from build123d import *

# Parameters (mm, degrees)
SKETCH1_W           = 45
SKETCH1_H           = 24
BOSS_EXTRUDE1_DEPTH = 9.3
SKETCH2_R           = 1.25
BOSS_EXTRUDE2_DEPTH = 9.3
SKETCH3_W           = 15
SKETCH3_H           = 24
BOSS_EXTRUDE3_DEPTH = 4.8
SKETCH4_W           = 11.1
SKETCH4_H           = 20.8
SKETCH4_R           = 0.75
CUT_EXTRUDE1_DEPTH  = 7


with BuildPart() as part:
    # Sketch1 → Boss-Extrude1 (new body)
    with BuildSketch(Plane(origin=(0, 0, 0), x_dir=(1, 0, 0), z_dir=(0, 1, 0))):
        with Locations((22.5, 12)):
            Rectangle(SKETCH1_W, SKETCH1_H)
    extrude(amount=BOSS_EXTRUDE1_DEPTH)

    # Sketch2 → Boss-Extrude2 (add)
    with BuildSketch(Plane(origin=(45, 0, 0), x_dir=(0, 0, -1), z_dir=(1, 0, 0))):
        with Locations((12, 2.083449871)):
            Circle(SKETCH2_R)
    extrude(amount=BOSS_EXTRUDE2_DEPTH)

    # Sketch3 → Boss-Extrude3 (add)
    with BuildSketch(Plane(origin=(0, 9.3, 0), x_dir=(1, 0, 0), z_dir=(0, 1, 0))):
        with Locations((7.5, 12)):
            Rectangle(SKETCH3_W, SKETCH3_H)
    extrude(amount=BOSS_EXTRUDE3_DEPTH)

    # Sketch4 → Cut-Extrude1 (cut)
    with BuildSketch(Plane(origin=(0, 14.1, 0), x_dir=(1, 0, 0), z_dir=(0, 1, 0))):
        with Locations((7.85, 12)):
            Rectangle(SKETCH4_W, SKETCH4_H)
        with Locations((4.85, 19.9)):
            Circle(SKETCH4_R, mode=Mode.SUBTRACT)
        with Locations((7.85, 19.9)):
            Circle(SKETCH4_R, mode=Mode.SUBTRACT)
        with Locations((10.85, 19.9)):
            Circle(SKETCH4_R, mode=Mode.SUBTRACT)
        with Locations((4.85, 17.3)):
            Circle(SKETCH4_R, mode=Mode.SUBTRACT)
        with Locations((7.85, 17.3)):
            Circle(SKETCH4_R, mode=Mode.SUBTRACT)
        with Locations((10.85, 17.3)):
            Circle(SKETCH4_R, mode=Mode.SUBTRACT)
        with Locations((4.85, 14.7)):
            Circle(SKETCH4_R, mode=Mode.SUBTRACT)
        with Locations((7.85, 14.7)):
            Circle(SKETCH4_R, mode=Mode.SUBTRACT)
        with Locations((10.85, 14.7)):
            Circle(SKETCH4_R, mode=Mode.SUBTRACT)
        with Locations((4.85, 12.1)):
            Circle(SKETCH4_R, mode=Mode.SUBTRACT)
        with Locations((7.85, 12.1)):
            Circle(SKETCH4_R, mode=Mode.SUBTRACT)
        with Locations((10.85, 12.1)):
            Circle(SKETCH4_R, mode=Mode.SUBTRACT)
        with Locations((4.85, 9.5)):
            Circle(SKETCH4_R, mode=Mode.SUBTRACT)
        with Locations((7.85, 9.5)):
            Circle(SKETCH4_R, mode=Mode.SUBTRACT)
        with Locations((10.85, 9.5)):
            Circle(SKETCH4_R, mode=Mode.SUBTRACT)
        with Locations((4.85, 6.9)):
            Circle(SKETCH4_R, mode=Mode.SUBTRACT)
        with Locations((7.85, 6.9)):
            Circle(SKETCH4_R, mode=Mode.SUBTRACT)
        with Locations((10.85, 6.9)):
            Circle(SKETCH4_R, mode=Mode.SUBTRACT)
        with Locations((4.85, 4.3)):
            Circle(SKETCH4_R, mode=Mode.SUBTRACT)
        with Locations((7.85, 4.3)):
            Circle(SKETCH4_R, mode=Mode.SUBTRACT)
        with Locations((10.85, 4.3)):
            Circle(SKETCH4_R, mode=Mode.SUBTRACT)
    extrude(amount=-CUT_EXTRUDE1_DEPTH, mode=Mode.SUBTRACT)


solid = part.part
Design review of the part built by this model. Coordinates are the model's own, in mm. A direction names the side the tool comes from. Coordinates: 2 decimals unless noted, no trailing zeros. Order: outer loops, then holes, each group sorted by start corner. A loop starts at its lowest first (then second) coordinate and runs counter-clockwise, first axis right, second up.
Item 1: Take a section at D-D, the plane x = 40. Write out the cut boundary in (y, z), then the cut area to 3 significant figures.
Item 2: Take a section at B-B, the plane z = -6.9. Write out the cut boundary in (x, y), then the cut area to 3 significant figures.
Item 3: Take a section at C-C, the plane y = 4.75. Write out the cut boundary in (x, z), then the cut area to 3 significant figures.
Item 4: For faces 1 (the flat face through (8, 14.1, -15)), 2 (the cylindrical face through (4.752, 10.649, -10.244)), 3 (the flat face through (15, 12, -12)), list the 3-axis set-ups (+Z, -Z, +X, -X, +Y, -Y) from which the entire face can be reached by the end or side of a thin tool; tool diameter is ignored.
Item 5: Take a section at A-A, the plane y = 8. Count the separate pieces of the cut face and the enclosed holes in it, then the cut area to 3 significant figures.
Item 6: The part is to be moulded in two halves that separate along Z. For faces 4 (the cylindrical face through (4.752, 10.649, -20.644)), 5 (the flat face through (22, 5, -24)), 6 (the cylindrical face through (7.687, 10.649, -13.968)), 7 (the flat face through (11, 14.1, -12)), say which applies: pulls with the +Z half, pulls with the -Z half, needs draft (parallel to the pull), parting line crosses it, or undercut.
Item 7: For line 1 (X direction, y = 13.25, z = -16.25); line 2 (X direction, y = 4.75, z = -20.25); line 3 (Y direction, x = 10, z = -13.25), list the stretches that pass through material, from the lowest coordinate up.
Item 8: For pin 1 Ø2 at (y, z) = (2.5, -21) entering from +X; pin 2 Ø2 at (x, z) = (43, -16.5) entering from +Y, all flat-tipped, find the tip position at first contact; note any pin that passes through.
The answers:
1. outline: (0, -24) - (9.3, -24) - (9.3, 0) - (0, 0) - close
1. area: 223 mm2
2. outline: (0, 0) - (45, 0) - (45, 9.3) - (15, 9.3) - (15, 14.1) - (13.4, 14.1) - (13.4, 7.1) - (11.6, 7.1) - (11.6, 14.1) - (10.1, 14.1) - (10.1, 7.1) - (8.6, 7.1) - (8.6, 14.1) - (7.1, 14.1) - (7.1, 7.1) - (5.6, 7.1) - (5.6, 14.1) - (4.1, 14.1) - (4.1, 7.1) - (2.3, 7.1) - (2.3, 14.1) - (0, 14.1) - close
2. area: 444 mm2
3. outline: (0, -24) - (45, -24) - (45, 0) - (0, 0) - close
3. area: 1,080 mm2
4. face 1: +Z, -Z, +X, -X, +Y
4. face 2: +Y
4. face 3: +Z, -Z, +X, +Y
5. separate pieces: 22
5. enclosed holes: 1
5. area: 886 mm2
6. face 4: undercut
6. face 5: pulls with the -Z half
6. face 6: undercut
6. face 7: needs draft
7. line 1: x = 0 to 2.3, 13.4 to 15
7. line 2: x = 0 to 45
7. line 3: y = 0 to 7.1
8. pin 1: stops at x = 45
8. pin 2: stops at y = 9.3
